Work out the finished part from the listing and answer in its coordinate system (mm). Face numbers are marked on the shaded views. A direction names the side the tool comes from. Round coordinates to 2 decimals unless told otherwise and drop trailing zeros. Order: outer loops, then holes, each group sorted by start corner. A loop starts at its lowest first (then second) coordinate and runs counter-clockwise, first axis right, second up. Notation, with made-up numbers: (81, 43) - (87, 43) arc R24 ccw to (87, 74) - close; hole circle Ø3 at (41.25, 27). An arc over 180 degrees is marked (long way). Answer in a Markdown table with one row per item.
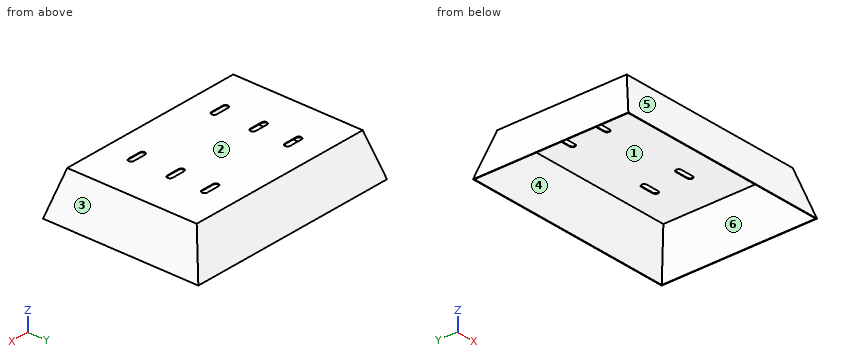
from build123d import *

# Parameters (mm, degrees)
F0_W     = 635
F0_H     = 457.2
F1_DEPTH = 127
F3_DEPTH = 457.201
F5_DEPTH = 330.2
F6_T     = -1.9304
F8_DEPTH = 127.001


with BuildPart() as f1:
    # F0 (on Top) → F1 (new body)
    with BuildSketch(Plane.XY):
        Rectangle(F0_W, F0_H)
    extrude(amount=F1_DEPTH)

    # F2 (on face) → F3 (cut, through all)
    with BuildSketch(Plane.XZ.offset(228.6)):
        Polygon((-317.5, 127), (-317.5, 0), (-279.4, 127), align=None)
        Polygon((279.4, 127), (317.5, 0), (317.5, 127), align=None)
    extrude(amount=-F3_DEPTH, mode=Mode.SUBTRACT)

    # F4 (on Right) → F5 (cut, symmetric)
    with BuildSketch(Plane.YZ):
        Polygon((-228.6, 127), (-228.6, 0), (-190.5, 127), align=None)
        Polygon((228.6, 0), (228.6, 127), (190.5, 127), align=None)
    extrude(amount=F5_DEPTH, both=True, mode=Mode.SUBTRACT)

    # F6
    f6_openings = [f1.faces().sort_by_distance(p)[0] for p in [
        (0, 0, 0),
    ]]
    offset(amount=F6_T, openings=f6_openings)

    # F7 (on face) → F8 (cut, through all)
    with BuildSketch(Plane.XY.offset(127)):
        with BuildLine():
            ThreePointArc((-158.75, 115.8875), (-166.6875, 107.95), (-158.75, 100.0125))
            Line((-158.75, 100.0125), (-120.65, 100.0125))
            ThreePointArc((-120.65, 100.0125), (-112.7125, 107.95), (-120.65, 115.8875))
            Line((-120.65, 115.8875), (-158.75, 115.8875))
        make_face()
        with BuildLine():
            ThreePointArc((158.75, 100.0125), (166.6875, 107.95), (158.75, 115.8875))
            Line((158.75, 115.8875), (120.65, 115.8875))
            ThreePointArc((120.65, 115.8875), (112.7125, 107.95), (120.65, 100.0125))
            Line((120.65, 100.0125), (158.75, 100.0125))
        make_face()
        with BuildLine():
            Line((120.65, -1.5875), (158.75, -1.5875))
            ThreePointArc((158.75, -1.5875), (166.6875, 6.35), (158.75, 14.2875))
            Line((158.75, 14.2875), (120.65, 14.2875))
            ThreePointArc((120.65, 14.2875), (112.7125, 6.35), (120.65, -1.5875))
        make_face()
        with BuildLine():
            Line((-158.75, -1.5875), (-120.65, -1.5875))
            ThreePointArc((-120.65, -1.5875), (-112.7125, 6.35), (-120.65, 14.2875))
            Line((-120.65, 14.2875), (-158.75, 14.2875))
            ThreePointArc((-158.75, 14.2875), (-166.6875, 6.35), (-158.75, -1.5875))
        make_face()
        with BuildLine():
            ThreePointArc((-158.75, -100.0125), (-166.6875, -107.95), (-158.75, -115.8875))
            Line((-158.75, -115.8875), (-120.65, -115.8875))
            ThreePointArc((-120.65, -115.8875), (-112.7125, -107.95), (-120.65, -100.0125))
            Line((-120.65, -100.0125), (-158.75, -100.0125))
        make_face()
        with BuildLine():
            ThreePointArc((120.65, -100.0125), (112.7125, -107.95), (120.65, -115.8875))
            Line((120.65, -115.8875), (158.75, -115.8875))
            ThreePointArc((158.75, -115.8875), (166.6875, -107.95), (158.75, -100.0125))
            Line((158.75, -100.0125), (120.65, -100.0125))
        make_face()
    extrude(amount=-F8_DEPTH, mode=Mode.SUBTRACT)


solid = f1.part
1) Which of the six approach directions +Z, -Z, +X, -X, +Y, -Y give full straight-line access (tool end or side, diameter ignored) to the marked faces 1 and 2?
Filled in:
| item | result |
|---|---|
| face 1 | -Z |
| face 2 | +Z, +X, -X, +Y, -Y |
2) Find section B-B, the plane z = 46.5. Give the vertices of the cut face in (x, y).
Filled in:
| item | result |
|---|---|
| outline | (-303.55, -214.65) - (303.55, -214.65) - (303.55, 214.65) - (-303.55, 214.65) - close; hole (-301.53, -212.63) - (301.53, -212.63) - (301.53, 212.63) - (-301.53, 212.63) - close |
3) Each of these flat-tipped pins is pushed along its axis until it touches: pin 1 (6 mm diameter, centred on x = 153.5, y = 113.5, fed in from -Z); pin 2 (1.5 mm diameter, centred on x = -130.5, z = 126, fed in from -Y) (3 decimals); pin 3 (8 mm diameter, centred on x = 123.5, z = 70, fed in from -Y). Where does it stop, or does it pass through?
Filled in:
| item | result |
|---|---|
| pin 1 | stops at z = 125.07 |
| pin 2 | stops at y = -191.025 |
| pin 3 | stops at y = -208.8 |
4) Find section A-A, the plane y = 6.35. Give the vertices of the cut face in (x, z), then the cut area to 3 significant figures.
Filled in:
| item | result |
|---|---|
| outline | (-317.5, 0) - (-315.48, 0) - (-277.96, 125.07) - (-166.69, 125.07) - (-166.69, 127) - (-279.4, 127) - close; (-112.71, 125.07) - (112.71, 125.07) - (112.71, 127) - (-112.71, 127) - close; (166.69, 125.07) - (277.96, 125.07) - (315.48, 0) - (317.5, 0) - (279.4, 127) - (166.69, 127) - close |
| area | 1,380 mm^2 |
5) Find section D-D, the plane z = 109.5. Give the vertices of the cut face in (x, y), then the cut area to 3 significant figures.
Filled in:
| item | result |
|---|---|
| outline | (-284.65, -195.75) - (284.65, -195.75) - (284.65, 195.75) - (-284.65, 195.75) - close; hole (-282.63, -193.73) - (282.63, -193.73) - (282.63, 193.73) - (-282.63, 193.73) - close |
| area | 3,860 mm^2 |
6) The mould has two halves that part along Y. Classify the marked faces 3, 4, 5 and 6: released by +Y, released by -Y, zero draft, split by the parting line, or undercut.
Filled in:
| item | result |
|---|---|
| face 3 | zero draft |
| face 4 | undercut |
| face 5 | released by -Y |
| face 6 | undercut |
7) Find section C-C, the plane x = 82. Give the vertices of the cut face in (y, z), then the cut area to 3 significant figures.
Filled in:
| item | result |
|---|---|
| outline | (-228.6, 0) - (-226.58, 0) - (-189.06, 125.07) - (189.06, 125.07) - (226.58, 0) - (228.6, 0) - (190.5, 127) - (-190.5, 127) - close |
| area | 1,240 mm^2 |
8) Find the intervals of material crossed by probe 1 along Y at (x, z) = (208, 111); probe 2 along X at (y, z) = (173, 115.5); probe 3 along Y at (x, z) = (-263.5, 89), in increasing order. Write a range as from..to.
Filled in:
| item | result |
|---|---|
| probe 1 | y = -195.3..-193.28, 193.28..195.3 |
| probe 2 | x = -282.85..-280.83, 280.83..282.85 |
| probe 3 | y = -201.9..-199.88, 199.88..201.9 |
